Autodesk Inventor part; units mm, degrees
ref_plane "WorkPlane1" through (0, 0, 0) normal (0, 0, 1) x (1, 0, 0)
ref_plane "MSC_PF1" through (0, 0, 0) normal (1, 0, 0) x (0, 1, 0)
ref_plane "MSC_PT1" through (0, 0, 0) normal (0, 0, -1) x (-1, 0, 0)
ref_plane "WorkPlane1" through (0, 0, 0) normal (0, 0, 1) x (1, 0, 0)
sketch "Sketch1" plane through (0, 0, 0) normal (0, 0, 1) x (1, 0, 0)
  point P0 (0, 0)
sketch "Sketch2" plane through (0, 0, 0) normal (0, 0, 1) x (1, 0, 0)
  line L0 (-8, 4.6189) -> (-8, -4.6189)
  line L1 (0, 9.2375) -> (-8, 4.6189)
  line L2 (8, 4.6189) -> (0, 9.2375)
  line L3 (8, -4.6189) -> (8, 4.6189)
  line L4 (0, -9.2375) -> (8, -4.6189)
  line L5 (-8, -4.6189) -> (0, -9.2375)
  circle A0 centre (0, 0) radius 8 construction
  dimension "d1" = 16
  dimension "d29" = 0
  dimension "d30" = 0
extrude "Extrusion1" add sketch "Sketch2" along normal blind 6.4
sketch "Sketch3" plane through (0, 0, 0) normal (1, 0, 0) x (0, 1, 0)
  line L0 (8, 6.4) -> (9.3375, 6.4)
  line L1 (9.3375, 5.6278) -> (8, 6.4)
  line L2 (9.3375, 6.4) -> (9.3375, 5.6278)
  line L3 (0, -1.28) -> (0, 7.68)
  line L4 (9.2375, 0) -> (9.2375, 6.4)
  dimension "d25" = 0.1
  dimension "d26" = 0
  dimension "d27" = 60
  dimension "d28" = 8
revolve "Revolution1" cut sketch "Sketch3" angle 360 about axis through (0, 0, -10) along (0, 0, 1)
sketch "Sketch4" plane through (0, 0, 0) normal (1, 0, 0) x (0, 1, 0)
  line L0 (0, -20) -> (0, 0)
  line L1 (-5, -20) -> (0, -20)
  line L2 (-5, 0) -> (-5, -20)
  line L3 (0, 0) -> (-5, 0)
  line L4 (0, -20) -> (0, 0)
  line L5 (-6, 0) -> (1, 0)
  line L6 (0, -24) -> (0, 4)
  dimension "d18" = 5
  dimension "d20" = 20
  dimension "d33" = 0
  dimension "d34" = 0
revolve "Revolution2" add sketch "Sketch4" angle 360 about axis through (0, 0, -20) along (0, 0, -1)
chamfer "Chamfer1" distance 0.75 angle 45 1 edges at (0, 5, -20)
fillet "Fillet1" radius 0.4 1 edges at (0, 5, 0)
thread "Thread1"
ref_plane "MSC_PF1" through (0, 0, 0) normal (1, 0, 0) x (0, 1, 0)
ref_plane "MSC_PT1" through (0, 0, 0) normal (0, 0, -1) x (-1, 0, 0)
equation "\"d22\" = 0.5 * PTC"
equation "\"d23\" = 0.5 * PTC"
equation "\"d24\" = r"
equation "\"d1\" = ParS"
equation "\"d6\" = ParK"
equation "\"b\" = NLG - 2 * PTC"
equation "\"d28\" = 0.5 * ParS"
equation "\"d18\" = 0.5 * NND"
equation "\"d20\" = NLG"
equation "\"NLG\" = 20"
equation "\"PTC\" = 1.5"
equation "\"ParK\" = 6.4"
equation "\"ParS\" = 16"
equation "\"msp_es\" = 0.577367 * ParS"
equation "\"r\" = 0.4"
properties part number "ISO 4018 - M10 x 20" material "Steel"
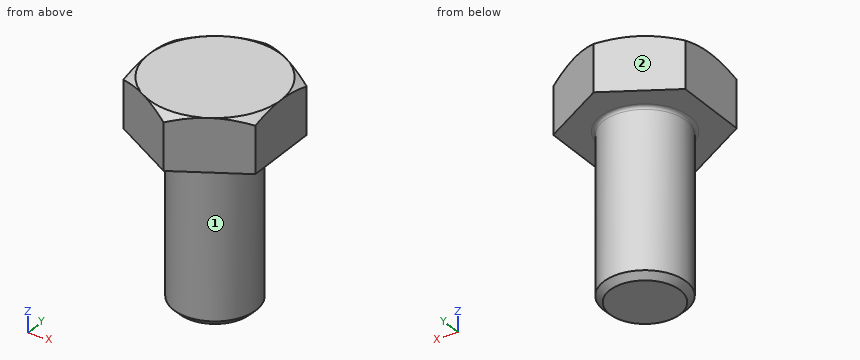
Part model, mm, in its own coordinate system. Face numbers are marked on the shaded views. A direction names the side the tool comes from. Give positions to 0.01 mm unless a question says otherwise; leave off trailing zeros. Write each loop counter-clockwise with the first axis right and the second up, starting at its lowest first coordinate (ties: lowest second). Pieces come first, ordered by that corner, then holes. Notation, with made-up numbers: M -13.75,30.25 L 6.25,30.25 A26 cw 6.25,57.25 Z; hole C 89,88.5 d6. An arc over 180 degrees is marked long. Use CSV: the item, a comma, the result in double quotes.
Item 1: Drill centre lines: probe 1 along Z at (x, y) = (5.25, -1); probe 2 along X at (y, z) = (3, -8.25); probe 3 along Y at (x, z) = (-6.25, 0.75). Where is each one in solid material? Low to high.
Taken from the geometry:
probe 1,"z = 0 to 6.4"
probe 2,"x = -4 to 4"
probe 3,"y = -5.63 to 5.63"
Item 2: Which spindle directions (+Z, -Z, +X, -X, +Y, -Y) get a long thin tool onto all of the face, cutting with end or side? Do the marked faces 1 and 2. Say none if no direction does.
Taken from the geometry:
face 1,"-Z"
face 2,"+Z, -Z, -X, +Y"
Item 3: Pin check, flat tips, straight feed: P1, Ø6, axis at x = -3, z = -3.5, coming from the +Y side; P2, Ø4, axis at x = 3, z = -11, coming from the -Y side. Stop position of each tip, or through.
Taken from the geometry:
P1,"stops at y = 5"
P2,"stops at y = -4.9"
Item 4: Slice it at A-A on z = -16. Write the cut outline in (x, y), plus the area to 3 significant figures.
Taken from the geometry:
outline,"C 0,0 d10"
area,"78.5 mm²"
